Input: part model. Units: mm. Frame: model coordinates. A direction names the side the tool comes from. Round coordinates to 2 decimals unless told otherwise and drop trailing zeros. Order: outer loops, then holes, each group sorted by start corner. A loop starts at its lowest first (then second) coordinate and runs counter-clockwise, first axis right, second up. Notation, with made-up numbers: (40, 66) -> (86, 66) arc R27 ccw to (86, 86) -> close; hole circle Ø9 at (-23.5, 78). An arc over 180 degrees is marked (long way). Answer as CSV lines item,"result". Start each with the question number.
1) Section query B-B, the plane z = 12.7. Output: boundary loops of the cut face in (x, y).
2) Access query for faces 4 (the face through (0, 25, 328.383)), 5 (the face through (3.414, -0.444, 18.054)), 6 (the face through (0, -25, 328.383)), 7 (the face through (19.05, 0, 241)), 8 (the face through (-19.856, 18.208, 672.211)). Directions: +Z, -Z, +X, -X, +Y, -Y. A direction counts if a zero-diameter tool reaches every point of the face in a straight line with its end or side. Return the directions, or none.
3) Line query: L1, parallel to Z at x = 0, y = -14; L2, parallel to Z at x = -1, y = 0; L3, parallel to Z at x = -3.5, y = -26. Output: solid intervals per line, ascending.
4) Section query C-C, the plane y = 0. Output: boundary loops of the cut face in (x, z), and give its area (3 significant figures).
5) First-contact query: P1, Ø4, axis at y = 5.5, z = 656.5, coming from the +X side; P2, Ø6, axis at y = 19.5, z = 350.5, coming from the -X side; P3, Ø2, axis at x = 8, z = 591.5, coming from the +Y side. Flat tips, straight axial feed; report the tip coordinate or a pass-through.
6) Section query A-A, the plane x = 0. Output: boundary loops of the cut face in (y, z), and give its area (3 significant figures).
7) Section query D-D, the plane z = 238. Output: boundary loops of the cut face in (x, y).
8) Mould query, pull axis Z, two halves, no side actions, for faces 1 (the face through (0, 19.05, 467)), 2 (the face through (0, 0, 0)), 3 (the face through (-19.05, 0, 241)). Classes: +Z half, -Z half, draft (parallel to the pull), parting line (faces both ways), or undercut.
```python
from build123d import *

# Parameters (mm, degrees)
SKETCH2_W           = 38.1
SKETCH2_H           = 38.1
BOSS_EXTRUDE1_DEPTH = 609.6
SKETCH3_R           = 26.940768363
BOSS_EXTRUDE2_DEPTH = 127
CUT_EXTRUDE2_DEPTH  = 127
BOSS_EXTRUDE3_DEPTH = 38.1
SKETCH6_R           = 6.35
CUT_EXTRUDE4_DEPTH  = 64.5
SKETCH7_R           = 6.35
CUT_EXTRUDE5_DEPTH  = 533.4


with BuildPart() as part:
    # Sketch2 → Boss-Extrude1 (new body)
    with BuildSketch(Plane.XY):
        Rectangle(SKETCH2_W, SKETCH2_H)
    extrude(amount=BOSS_EXTRUDE1_DEPTH)

    # Sketch3 → Boss-Extrude2 (add)
    with BuildSketch(Plane.XY.offset(609.6)):
        Circle(SKETCH3_R)
    extrude(amount=BOSS_EXTRUDE2_DEPTH)

    # Sketch4 → Cut-Extrude2 (cut)
    with BuildSketch(Plane.XZ.offset(19.05)):
        with BuildLine():
            ThreePointArc((-6.35, 152.4), (0, 146.05), (6.35, 152.4))
            Line((6.35, 152.4), (-6.35, 152.4))
        make_face()
        with BuildLine():
            Line((-6.35, 152.4), (6.35, 152.4))
            ThreePointArc((6.35, 152.4), (0, 158.75), (-6.35, 152.4))
        make_face()
    extrude(amount=-CUT_EXTRUDE2_DEPTH, mode=Mode.SUBTRACT)

    # Sketch5 → Boss-Extrude3 (add)
    with BuildSketch(Plane(origin=(19.05, 0, 0), x_dir=(0, 0, -1), z_dir=(1, 0, 0))):
        Polygon((0, 0), (0, 31.75), (-328.383343368, 31.75), (-328.383343368, -31.75), (0, -31.75), align=None)
    extrude(amount=-BOSS_EXTRUDE3_DEPTH)

    # Sketch6 → Cut-Extrude4 (cut, through all)
    with BuildSketch(Plane.XZ.offset(31.75)):
        with Locations((0, 152.494180782)):
            Circle(SKETCH6_R)
    extrude(amount=-CUT_EXTRUDE4_DEPTH, mode=Mode.SUBTRACT)

    # Sketch7 → Cut-Extrude5 (cut)
    with BuildSketch(Plane.XZ.offset(31.75)):
        with Locations((0, 12.7)):
            Circle(SKETCH7_R)
    extrude(amount=-CUT_EXTRUDE5_DEPTH, mode=Mode.SUBTRACT)


solid = part.part
```
Findings:
1,outline,"(-19.05, -31.75) -> (-6.35, -31.75) -> (-6.35, 31.75) -> (-19.05, 31.75) -> close; (6.35, -31.75) -> (19.05, -31.75) -> (19.05, 31.75) -> (6.35, 31.75) -> close"
2,face 4,"+X, -X, +Y"
2,face 5,"+Y, -Y"
2,face 6,"+X, -X, -Y"
2,face 7,"-Z, +X, +Y, -Y"
2,face 8,"+Z"
3,L1,"z = 0 to 6.35, 19.05 to 146.14, 158.84 to 736.6"
3,L2,"z = 0 to 6.43, 18.97 to 146.22, 158.76 to 736.6"
3,L3,"z = 0 to 7.4, 18 to 147.2, 157.79 to 328.38, 609.6 to 736.6"
4,outline,"(-26.94, 609.6) -> (-19.05, 609.6) -> (-19.05, 0) -> (19.05, 0) -> (19.05, 609.6) -> (26.94, 609.6) -> (26.94, 736.6) -> (-26.94, 736.6) -> close; hole circle Ø12.7 at (0, 12.7); hole circle Ø12.7 at (0, 152.49)"
4,area,"29,800 mm^2"
5,P1,"stops at x = 26.71"
5,P2,"stops at x = -19.05"
5,P3,"stops at y = 19.05"
6,outline,"(-31.75, 0) -> (31.75, 0) -> (31.75, 6.35) -> (-31.75, 6.35) -> close; (-31.75, 19.05) -> (31.75, 19.05) -> (31.75, 146.14) -> (-31.75, 146.14) -> close; (-31.75, 158.84) -> (31.75, 158.84) -> (31.75, 328.38) -> (19.05, 328.38) -> (19.05, 609.6) -> (26.94, 609.6) -> (26.94, 736.6) -> (-26.94, 736.6) -> (-26.94, 609.6) -> (-19.05, 609.6) -> (-19.05, 328.38) -> (-31.75, 328.38) -> close"
6,area,"36,800 mm^2"
7,outline,"(-19.05, -31.75) -> (19.05, -31.75) -> (19.05, 31.75) -> (-19.05, 31.75) -> close"
8,face 1,"undercut"
8,face 2,"-Z half"
8,face 3,"draft"
